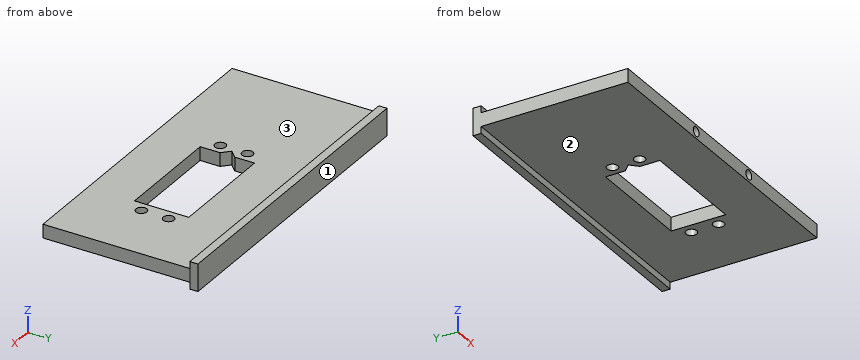
from build123d import *

# Parameters (mm, degrees)
SKETCH_1_W          = 115
SKETCH_1_H          = 54
SKETCH_1_R          = 2
SKETCH_1_W_2        = 40
SKETCH_1_H_2        = 20
EXTRUDE_3_DEPTH     = 5
SKETCH_3_R          = 1.75
CUT_EXTRUDE_2_DEPTH = 15
CUT_EXTRUDE_3_DEPTH = 10
EXTRUDE_4_DEPTH     = 3


with BuildPart() as part:
    # 草圖1 → 填料-伸長3 (new body)
    with BuildSketch(Plane.XY):
        with Locations((13.062480584, -3.484099434)):
            Rectangle(SKETCH_1_W, SKETCH_1_H)
        with Locations((-0.937519416, -8.484099434)):
            Circle(SKETCH_1_R, mode=Mode.SUBTRACT)
        with Locations((47.062480584, -8.484099434)):
            Circle(SKETCH_1_R, mode=Mode.SUBTRACT)
        with Locations((-0.937519416, 1.515900566)):
            Circle(SKETCH_1_R, mode=Mode.SUBTRACT)
        with Locations((47.062480584, 1.515900566)):
            Circle(SKETCH_1_R, mode=Mode.SUBTRACT)
        with Locations((23.062480584, -3.484099434)):
            Rectangle(SKETCH_1_W_2, SKETCH_1_H_2, mode=Mode.SUBTRACT)
    extrude(amount=EXTRUDE_3_DEPTH)

    # 草圖3 → 除料-伸長2 (cut)
    with BuildSketch(Plane.XZ.offset(30.484099434)):
        with Locations(Location((29.062480584, 2.5, 0), (0, 0, 270))):
            Circle(SKETCH_3_R)
        with Locations(Location((-2.937519416, 2.5, 0), (0, 0, 270))):
            Circle(SKETCH_3_R)
    extrude(amount=-CUT_EXTRUDE_2_DEPTH, mode=Mode.SUBTRACT)

    # 草圖4 → 除料-伸長3 (cut)
    with BuildSketch(Plane.XY.offset(5)):
        Polygon((0.340707034, -3.484099434), (3.062480584, -6.205872984), (3.062480584, -0.762325884), align=None)
    extrude(amount=-CUT_EXTRUDE_3_DEPTH, mode=Mode.SUBTRACT)

    # 草圖5 → 填料-伸長4 (add)
    with BuildSketch(Plane(origin=(0, 23.515900566, 0), x_dir=(1, 0, 0), z_dir=(0, 1, 0))):
        Polygon((-44.437519416, 0), (-44.437519416, 2.5), (70.560278635, 2.5), (70.560278635, -7.5), (-44.437519416, -7.5), align=None)
    extrude(amount=EXTRUDE_4_DEPTH)


solid = part.part
Geometry check sheet. Reference: the model listing, model coordinates, mm. Face numbers are marked on the shaded views. A direction names the side the tool comes from. Give positions to 0.01 mm unless a question says otherwise; leave off trailing zeros. Write each loop counter-clockwise with the first axis right and the second up, starting at its lowest first coordinate (ties: lowest second). Pieces come first, ordered by that corner, then holes. Notation, with made-up numbers: M 71.25,-7.5 L 125.25,-7.5 A31 ccw 125.25,23.5 Z; hole C 52,-16 d10. An arc over 180 degrees is marked long. One line per question, with ' | ' between items.
1. Cross-section at B-B (z = 2.5). Count the separate pieces of the cut face and the enclosed holes in it, plus the area to 3 significant figures.
Ans:
separate pieces: 1 | enclosed holes: 5 | area: 5,590 mm2
2. Cross-section at C-C (x = -29). Enter the section's corners in (y, z).
Ans:
outline: M -30.48,0 L 23.52,0 L 23.52,-2.5 L 26.52,-2.5 L 26.52,7.5 L 23.52,7.5 L 23.52,5 L -30.48,5 Z
3. Scan lines: line 1 along X through (y, z) = (-20.75, 2.5); line 2 along X through (y, z) = (-13, 3.75); line 3 along X through (y, z) = (-3.5, 4). Record each from-to range of solid material in increasing order. Write a range as from..to.
Ans:
line 1: -44.44..-4.69, -1.19..27.31, 30.81..70.56 | line 2: -44.44..3.06, 43.06..70.56 | line 3: -44.44..0.36, 43.06..70.56
4. Cross-section at D-D (y = -26). Enter the section's corners in (x, z), plus the area to 3 significant figures.
Ans:
outline: M -44.44,0 L 70.56,0 L 70.56,5 L -44.44,5 Z; hole C -2.94,2.5 d3.5; hole C 29.06,2.5 d3.5 | area: 556 mm2
5. Gauge pin test, flat ends, axial feed: pin 1 (10 mm diameter, centred on x = -24, y = -15, fed in from +Z); pin 2 (4 mm diameter, centred on x = 29, z = 2, fed in from -Y); pin 3 (6 mm diameter, centred on x = -28, y = 1, fed in from -Z); pin 4 (2 mm diameter, centred on x = 34, z = 6.5, fed in from -Y). Record the tip position at first contact, or that the pin passes through.
Ans:
pin 1: z = 5 | pin 2: y = -30.48 | pin 3: z = 0 | pin 4: y = 23.52
6. Cross-section at A-A (x = 19). Enter the section's corners in (y, z).
Ans:
outline: M -30.48,0 L -13.48,0 L -13.48,5 L -30.48,5 Z; M 6.52,0 L 23.52,0 L 23.52,-2.5 L 26.52,-2.5 L 26.52,7.5 L 23.52,7.5 L 23.52,5 L 6.52,5 Z
7. Set-up check for the marked faces 1, 2 and 3: record each of +Z, -Z, +X, -X, +Y, -Y from which the full face is reachable in a straight line by a thin tool's end or side.
Ans:
face 1: +Z, -Z, +X, -X, +Y | face 2: -Z, +X, -X, -Y | face 3: +Z, +X, -X, -Y
